Work out the finished part from the listing and answer in its coordinate system (mm). A direction names the side the tool comes from. Give positions to 0.01 mm unless a question says otherwise; leave off trailing zeros. Order: outer loops, then holes, each group sorted by start corner. A loop starts at its lowest first (then second) coordinate and runs counter-clockwise, first axis right, second up.
```python
from build123d import *

# Parameters (mm, degrees)
BOSS_EXTRUDE1_DEPTH = 3
SKETCH3_R           = 1
BOSS_EXTRUDE2_DEPTH = 3
SKETCH4_R           = 1
CUT_EXTRUDE1_DEPTH  = 3


with BuildPart() as part:
    # Sketch2 → Boss-Extrude1 (new body)
    with BuildSketch(Plane.XY):
        with BuildLine():
            Line((-36.5050045, 13.800340042), (-28.969106115, 13.800340042))
            ThreePointArc((-28.969106115, 13.800340042), (-25.237055307, 12.800340042), (-28.969106115, 11.800340042))
            Line((-28.969106115, 11.800340042), (-36.5050045, 11.800340042))
            ThreePointArc((-36.5050045, 11.800340042), (-40.237055307, 12.800340042), (-36.5050045, 13.800340042))
        make_face()
    extrude(amount=BOSS_EXTRUDE1_DEPTH)

    # Sketch3 → Boss-Extrude2 (add)
    with BuildSketch(Plane.XY.offset(3)):
        with Locations((-38.237055307, 12.800340042)):
            Circle(SKETCH3_R)
    extrude(amount=BOSS_EXTRUDE2_DEPTH)

    # Sketch4 → Cut-Extrude1 (cut)
    with BuildSketch(Plane(origin=(0, 0, 0), x_dir=(-1, 0, 0), z_dir=(0, 0, -1))):
        with Locations((27.237055307, 12.800340042)):
            Circle(SKETCH4_R)
    extrude(amount=-CUT_EXTRUDE1_DEPTH, mode=Mode.SUBTRACT)


solid = part.part
```
1. Given P1, Ø1.2, axis at x = -29, y = 12.5, coming from the +Z side; P2, Ø1.5, axis at x = -31, z = 3.5, coming from the -Y side; P3, Ø3.5, axis at x = -31, z = 1, coming from the +Y side, each flat-ended and moving along its own axis, determine where each tip first touches the part or whether it passes through.
Findings below:
P1: stops at z = 3
P2: stops at y = 11.8
P3: stops at y = 13.8
2. Straight lines are drawn through the part: probe 1 along Y at (x, z) = (-33.75, 0.8); probe 2 along Z at (x, y) = (-37, 12.95); probe 3 along X at (y, z) = (14.15, 2.25). For each, find the intervals that lie inside material, in ascending order.
Findings below:
probe 1: y = 11.8 to 13.8
probe 2: z = 0 to 3
probe 3: x = -39.71 to -36.76, -28.71 to -25.76
3. The part is cut by section D-D (x = -32.75). Write down the section's boundary in (y, z).
Findings below:
outline: (11.8, 0) - (13.8, 0) - (13.8, 3) - (11.8, 3) - close
4. The part is cut by section A-A (y = 12.35). Write down the section's boundary in (x, z).
Findings below:
outline: (-40.19, 0) - (-28.13, 0) - (-28.13, 3) - (-37.34, 3) - (-37.34, 6) - (-39.13, 6) - (-39.13, 3) - (-40.19, 3) - close; (-26.34, 0) - (-25.29, 0) - (-25.29, 3) - (-26.34, 3) - close
5. The mould has two halves that part along Y. Classify faces 4 (the face through (-40.236, 12.727, 1.479)), 5 (the face through (-33, 11.8, 1)), 6 (the face through (-27.02, 11.824, 1.479)): pulls with the +Y half, pulls with the -Y half, needs draft (parallel to the pull), parting line crosses it, or undercut.
Findings below:
face 4: parting line crosses it
face 5: pulls with the -Y half
face 6: undercut
6. Which of the six approach directions +Z, -Z, +X, -X, +Y, -Y give full straight-line access (tool end or side, diameter ignored) to faces 1 (the face through (-37.313, 12.417, 4.479)), 2 (the face through (-25.24, 12.87, 1.48)), 3 (the face through (-33, 13.8, 1))?
Findings below:
face 1: +Z
face 2: +Z, -Z
face 3: +Z, -Z, +Y
7. The part is cut by section B-B (x = -27.5). Write down the section's boundary in (y, z).
Findings below:
outline: (10.82, 0) - (11.84, 0) - (11.84, 3) - (10.82, 3) - close; (13.77, 0) - (14.78, 0) - (14.78, 3) - (13.77, 3) - close
8. The part is cut by section C-C (z = 0.65). Write down the section's boundary in (x, y) (3 decimals), then the cut area to 3 significant figures.
Findings below:
outline: (-36.505, 11.8) - (-28.969, 11.8) arc R2 ccw (long way) to (-28.969, 13.8) - (-36.505, 13.8) arc R2 ccw (long way) to start; hole circle Ø2 at (-27.237, 12.8)
area: 36.3 mm2
